Verification items for the finished model (mm, model axes). A direction names the side the tool comes from. Round coordinates to 2 decimals unless told otherwise and drop trailing zeros. Order: outer loops, then holes, each group sorted by start corner. A loop starts at its lowest first (then second) coordinate and runs counter-clockwise, first axis right, second up. Notation, with made-up numbers: (15, 5) -> (31, 5) arc R13 cw to (31, 10) -> close; hole circle Ø1 at (-18, 65). An arc over 180 degrees is marked (long way). Put each result on its own line as item: value.
```python
from build123d import *

# Parameters (mm, degrees)
SKETCH1_R           = 22.5
SKETCH1_R_2         = 20
BOSS_EXTRUDE1_DEPTH = 200
SKETCH2_R           = 32.5
SKETCH2_R_2         = 22.5
BOSS_EXTRUDE2_DEPTH = 5
SKETCH3_R           = 32.5
SKETCH3_R_2         = 22.5
BOSS_EXTRUDE3_DEPTH = 5


with BuildPart() as part:
    # Sketch1 → Boss-Extrude1 (new body, symmetric)
    with BuildSketch(Plane(origin=(0, 0, 0), x_dir=(1, 0, 0), z_dir=(0, 1, 0))):
        Circle(SKETCH1_R)
        Circle(SKETCH1_R_2, mode=Mode.SUBTRACT)
    extrude(amount=BOSS_EXTRUDE1_DEPTH, both=True)

    # Sketch2 → Boss-Extrude2 (add)
    with BuildSketch(Plane(origin=(0, 100, 0), x_dir=(1, 0, 0), z_dir=(0, 1, 0))):
        Circle(SKETCH2_R)
        Circle(SKETCH2_R_2, mode=Mode.SUBTRACT)
    extrude(amount=BOSS_EXTRUDE2_DEPTH)

    # Sketch3 → Boss-Extrude3 (add)
    with BuildSketch(Plane(origin=(0, 0, 0), x_dir=(1, 0, 0), z_dir=(0, 1, 0))):
        Circle(SKETCH3_R)
        Circle(SKETCH3_R_2, mode=Mode.SUBTRACT)
    extrude(amount=-BOSS_EXTRUDE3_DEPTH)


solid = part.part
```
Item 1: Sectioned sample at B-B, the plane x = 0. Record the boundary of the cut face in (y, z), then the cut area to 3 significant figures.
Geometry check:
outline: (-200, -22.5) -> (-5, -22.5) -> (-5, -32.5) -> (0, -32.5) -> (0, -22.5) -> (100, -22.5) -> (100, -32.5) -> (105, -32.5) -> (105, -22.5) -> (200, -22.5) -> (200, -20) -> (-200, -20) -> close; (-200, 20) -> (200, 20) -> (200, 22.5) -> (105, 22.5) -> (105, 32.5) -> (100, 32.5) -> (100, 22.5) -> (0, 22.5) -> (0, 32.5) -> (-5, 32.5) -> (-5, 22.5) -> (-200, 22.5) -> close
area: 2,200 mm2
Item 2: Sectioned sample at A-A, the plane z = 0. Record the boundary of the cut face in (x, y).
Geometry check:
outline: (-32.5, -5) -> (-22.5, -5) -> (-22.5, -200) -> (-20, -200) -> (-20, 200) -> (-22.5, 200) -> (-22.5, 105) -> (-32.5, 105) -> (-32.5, 100) -> (-22.5, 100) -> (-22.5, 0) -> (-32.5, 0) -> close; (20, -200) -> (22.5, -200) -> (22.5, -5) -> (32.5, -5) -> (32.5, 0) -> (22.5, 0) -> (22.5, 100) -> (32.5, 100) -> (32.5, 105) -> (22.5, 105) -> (22.5, 200) -> (20, 200) -> close
Item 3: Sectioned sample at C-C, the plane y = 110.5. Record the boundary of the cut face in (x, z).
Geometry check:
outline: circle Ø45 at (0, 0); hole circle Ø40 at (0, 0)
Item 4: Material ranges on line 1 along Y through (x, z) = (23, 3); line 2 along X through (y, z) = (66.5, 0), recorded low to high.
Geometry check:
line 1: -5 to 0, 100 to 105
line 2: -22.5 to -20, 20 to 22.5
Item 5: Depth check by flat-ended pin: pin 1 Ø4 at (y, z) = (-54.5, 17.5) entering from -X; pin 2 Ø1.5 at (x, y) = (15, -85.5) entering from +Z; pin 3 Ø6 at (x, y) = (7.5, 47.5) entering from -Z. Enter the tip coordinate at first touch or a pass-through.
Geometry check:
pin 1: x = -16.31
pin 2: z = 17.41
pin 3: z = -22.05
Item 6: Tool access check on faces 4 (the face through (7, 0, -22)), 5 (the face through (10.382, -101.135, 19.961)), 6 (the face through (7, 105, -22)). Record the directions out of +Z, -Z, +X, -X, +Y, -Y that give a thin tool (end or side, any length) a straight path to the whole face; none if there is none.
Geometry check:
face 4: none
face 5: -Y
face 6: +Y
Item 7: Release check for a two-part mould opening along Y. For faces 1 (the face through (7, 100, -22)), 2 (the face through (10.382, 153.165, 19.961)), 3 (the face through (7, -5, -22)) record: pulls with the +Y half, pulls with the -Y half, needs draft (parallel to the pull), parting line crosses it, or undercut.
Geometry check:
face 1: undercut
face 2: needs draft
face 3: pulls with the -Y half
Item 8: Sectioned sample at D-D, the plane z = 27.5. Record the boundary of the cut face in (x, y).
Geometry check:
outline: (-17.32, -5) -> (17.32, -5) -> (17.32, 0) -> (-17.32, 0) -> close; (-17.32, 100) -> (17.32, 100) -> (17.32, 105) -> (-17.32, 105) -> close
